Drawing for the job (mm, zero at the part's lowest x, y, z). A direction names the side the tool comes from. Give positions to 0.01 mm unless a question says otherwise; leave off trailing zeros. Loops run counter-clockwise (first coordinate to the right, second up) from the corner with the lowest first, then second, coordinate; pieces in that order, holes last. Notation, with made-up numbers: (26, 88.5) -> (61, 88.5) arc R19 cw to (61, 122.5) -> close; hole circle Ø3 at (83, -5.5). An arc over 180 degrees is marked (long way). Write item = value, one per line.
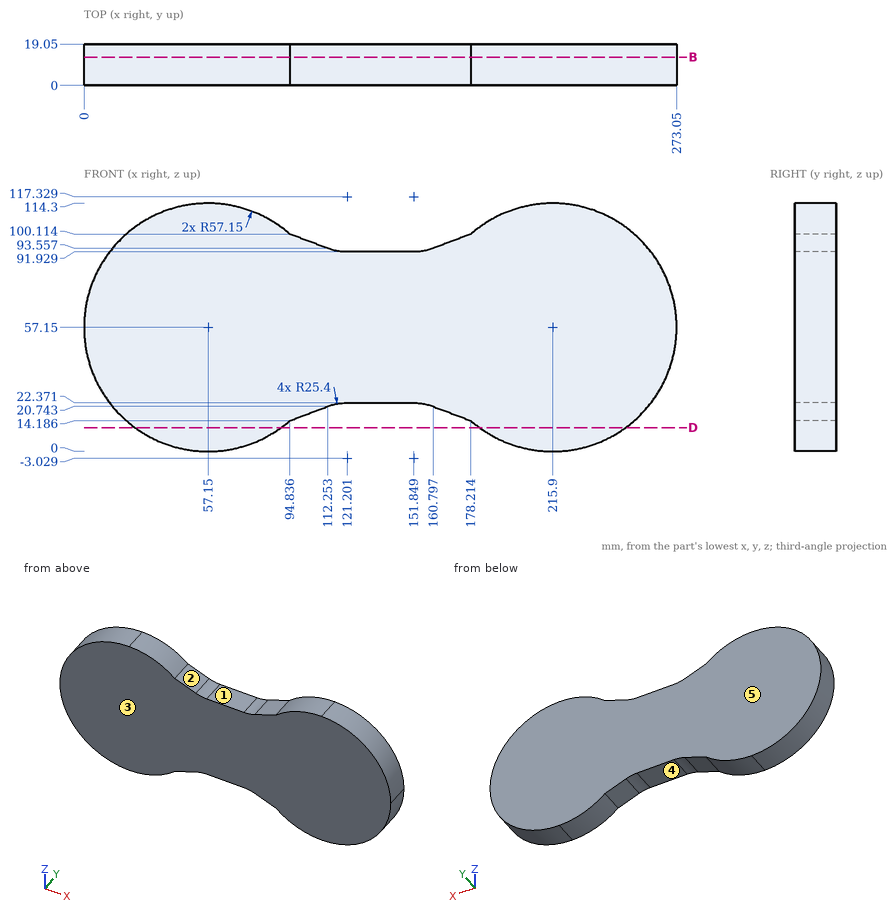
1) Which spindle directions (+Z, -Z, +X, -X, +Y, -Y) get a long thin tool onto all of the face, cutting with end or side? Do the marked faces 4 and 5. Say none if no direction does.
Resolved:
face_4 = -Z, +Y, -Y
face_5 = +Z, -Z, +X, -X, +Y
2) Pull direction X, two halves, no side cores. Call the marked faces 1, 2 and 3: pulls with the +X half, pulls with the -X half, needs draft (parallel to the pull), parting line crosses it, or undercut.
Resolved:
face_1 = undercut
face_2 = undercut
face_3 = needs draft
3) Slice it at D-D, the plane z = 11. List the corners of the cut face in (x, y).
Resolved:
outline = (23.44, 0) -> (90.86, 0) -> (90.86, 19.05) -> (23.44, 19.05) -> close; (182.19, 0) -> (249.61, 0) -> (249.61, 19.05) -> (182.19, 19.05) -> close
4) Drill centre lines: line 1 along Z through (x, y) = (144, 15); line 2 along X through (y, z) = (10, 7) (1 decimal); line 3 along Z through (x, y) = (116.5, 16.5). Where is each one in solid material? Low to high. Write a range as [from, to].
Resolved:
line_1 = [22.37, 91.93]
line_2 = [29.7, 84.6], [188.5, 243.3]
line_3 = [21.93, 92.37]
5) Slice it at B-B, the plane y = 13. List the corners of the cut face in (x, z).
Resolved:
outline = (94.84, 14.19) -> (112.25, 20.74) arc R25.4 cw to (121.2, 22.37) -> (151.85, 22.37) arc R25.4 cw to (160.8, 20.74) -> (178.21, 14.19) arc R57.15 ccw (long way) to (178.21, 100.11) -> (160.8, 93.56) arc R25.4 cw to (151.85, 91.93) -> (121.2, 91.93) arc R25.4 cw to (112.25, 93.56) -> (94.84, 100.11) arc R57.15 ccw (long way) to start
6) Drop flat-ended pins along their axis: P1, Ø4, axis at x = 154, y = 9, coming from the -Z side; P2, Ø5.5, axis at x = 143.5, y = 13.5, coming from the +Z side; P3, Ø1.5, axis at x = 70, y = 4.5, coming from the +Z side (1 decimal). Give the stop position or say it passes through.
Resolved:
P1 = 22.03
P2 = 91.93
P3 = 113
